Autodesk Inventor part; units mm, degrees
ref_plane "YZ Plane" through (0, 0, 0) normal (1, 0, 0) x (0, 1, 0)
ref_plane "XZ Plane" through (0, 0, 0) normal (0, 1, 0) x (-1, 0, 0)
ref_plane "XY Plane" through (0, 0, 0) normal (0, 0, 1) x (1, 0, 0)
sketch "Szkic1" plane through (0, 0, 0) normal (0, 1, 0) x (-1, 0, 0)
  line L0 (0, 0) -> (-45, 0)
  line L1 (-55, -10) -> (-55, -50)
  line L2 (-55, -50) -> (0, -50)
  line L3 (0, -50) -> (0, 0)
  arc A0 (-45, 0) -> (-55, -10) centre (-45, -10) ccw
  point P0 (-55, 0)
  dimension "d0" = 55
  dimension "d1" = 50
  dimension "d2" = 10
extrude "Wyciągnięcie proste1" add sketch "Szkic1" along normal blind 10
sketch "Szkic2" plane through (0, 10, 0) normal (0, 1, 0) x (1, 0, 0)
  line L0 (0, 50) -> (0, 0)
  line L1 (0, 50) -> (55, 50)
  line L2 (55, 50) -> (55, 30)
  line L3 (55, 30) -> (0, 30)
  line L4 (0, 30) -> (0, 50)
  dimension "d5" = 55
  dimension "d6" = 20
extrude "Wyciągnięcie proste2" add sketch "Szkic2" along normal blind 50
fillet "Zaokrąglenie1" radius 10 1 edges at (55, 60, -40)
sketch "Szkic3" plane through (0, 0, 0) normal (1, 0, 0) x (0, 1, 0)
  line L0 (0, -50) -> (0, 0)
  line L1 (0, 0) -> (10, 0)
  line L2 (10, -30) -> (10, 0)
  line L3 (10, -30) -> (60, -30)
  line L4 (60, -50) -> (60, -30)
  line L5 (0, -50) -> (60, -50)
  line L6 (60, -30) -> (50, -30)
  line L7 (10, -30) -> (60, -30)
  line L8 (10, -30) -> (50, -30)
  line L9 (60, -30) -> (10, 0)
sketch "Szkic4" plane through (0, 0, 0) normal (1, 0, 0) x (0, 1, 0)
  line L0 (60, -50) -> (60, -30)
  line L1 (10, -30) -> (50, -30)
  line L2 (60, -30) -> (10, -30)
  line L3 (10, -10) -> (10, 0)
  line L4 (10, -30) -> (10, 0)
  point P0 (0, 0)
extrude "Wyciągnięcie proste3" add sketch "Szkic3" along normal blind 10 contours L9 L3 L2
sketch "Szkic5" plane through (55, 10, -30) normal (0, 0, 1) x (1, 0, 0)
  line L0 (0, 0) -> (0, 40)
  line L1 (-45, 0) -> (-10, 0)
  point P0 (-55, -10)
  point P1 (-25, 30)
  dimension "d12" = 25
  dimension "d13" = 30
hole "Otwór1" at (30, 40, -30) direction (0, 0, -1) diameter 30 end through all
sketch "Szkic6" plane through (0, 10, 0) normal (0, 1, 0) x (1, 0, 0)
  line L0 (10, 30) -> (10, 0)
  line L1 (10, 30) -> (45, 30)
  point P0 (0, 0)
  point P1 (40, 15)
  point P2 (20, 15)
  dimension "d21" = 10
  dimension "d22" = 20
  dimension "d23" = 15
hole "Otwór2" at (20, 10, -15) at (40, 10, -15) direction (0, -1, 0) diameter 10 end through all
Work out the finished part from the listing and answer in its coordinate system (mm). A direction names the side the tool comes from. Round coordinates to 2 decimals unless told otherwise and drop trailing zeros. Write each loop counter-clockwise with the first axis right and the second up, starting at its lowest first coordinate (ties: lowest second). Pieces come first, ordered by that corner, then holes. Notation, with made-up numbers: (71, 23) - (99, 23) arc R17 cw to (99, 45) - close; hole circle Ø5 at (26, 21.5). An arc over 180 degrees is marked (long way). Return JSON: item names as keys, results as strings. Group by question number.
Q1. The part is cut by section D-D on x = 37.5. Write down the section's boundary in (y, z).
Q2. The part is cut by section C-C on x = 30. Write down the section's boundary in (y, z).
Q3. For faces 4 (the flat face through (10, 24, -21)), 5 (the flat face through (22, 5, 0)), determine the directions among +Z, -Z, +X, -X, +Y, -Y from which every point of the face is accessible in a straight line to the end or side of a thin tool.
Q4. Each of these flat-tipped pins is pushed along its axis until it touches: pin 1 Ø8 at (x, z) = (29.5, -20) entering from +Y; pin 2 Ø9 at (x, z) = (40, -15) entering from -Y; pin 3 Ø22.5 at (x, y) = (40, 29) entering from +Z. Where does it stop, or does it pass through?
Q5. Find the intervals of material crossed by L1, parallel to X at y = 4, z = -15; L2, parallel to Z at x = 20, y = 6; L3, parallel to Y at x = 30, z = -34, in increasing order.
Q6. The mould has two halves that part along Y. Classify faces 1 (the flat face through (33, 10, -15)), 2 (the cylindrical face through (35.043, 4.93, -15.651)), 3 (the cylindrical face through (29.34, 54.985, -40.14)): released by +Y, released by -Y, zero draft, split by the parting line, or undercut.
Q7. The part is cut by section B-B on y = 40. Write down the section's boundary in (x, z).
Q8. The part is cut by section A-A on z = -18. Write down the section's boundary in (x, y), then the cut area to 3 significant figures.
Solved:
{
 "1": {"outline": "(0, -50) - (27.01, -50) - (27.01, -30) - (10, -30) - (10, -19.33) - (0, -19.33) - close; (0, -10.67) - (10, -10.67) - (10, 0) - (0, 0) - close; (52.99, -50) - (60, -50) - (60, -30) - (52.99, -30) - close"},
 "2": {"outline": "(0, -50) - (25, -50) - (25, -30) - (10, -30) - (10, 0) - (0, 0) - close; (55, -50) - (60, -50) - (60, -30) - (55, -30) - close"},
 "3": {"face 4": "+Z, +X, +Y", "face 5": "+Z, +X, -X, +Y, -Y"},
 "4": {"pin 1": "y = 10", "pin 2": "through", "pin 3": "z = -30"},
 "5": {"L1": "0 to 15, 25 to 35, 45 to 55", "L2": "-50 to -20, -10 to 0", "L3": "0 to 25, 55 to 60"},
 "6": {"face 1": "released by +Y", "face 2": "zero draft", "face 3": "undercut"},
 "7": {"outline": "(0, -50) - (15, -50) - (15, -30) - (10, -30) - (10, -18) - (0, -18) - close; (45, -50) - (55, -50) - (55, -30) - (45, -30) - close"},
 "8": {"outline": "(0, 0) - (16, 0) - (16, 10) - (10, 10) - (10, 40) - (0, 40) - close; (24, 0) - (36, 0) - (36, 10) - (24, 10) - close; (44, 0) - (55, 0) - (55, 10) - (44, 10) - close", "area": "690 mm²"}
}
